from build123d import *

# Parameters (mm, degrees)
SKETCH1_R           = 5.08
BOSS_EXTRUDE1_DEPTH = 20.8
SKETCH2_R           = 10.16
BOSS_EXTRUDE2_DEPTH = 13.97
SKETCH4_R           = 6.052157879
SKETCH3_R           = 6.450000054
CHAMFER1_SIZE       = 5.08


with BuildPart() as part:
    # Sketch1 → Boss-Extrude1 (new body)
    with BuildSketch(Plane(origin=(0, 0, 0), x_dir=(1, 0, 0), z_dir=(0, 1, 0))):
        with Locations(Location((0, 0, 0), (0, 0, 270))):
            Circle(SKETCH1_R)
    extrude(amount=BOSS_EXTRUDE1_DEPTH)

    # Sketch2 → Boss-Extrude2 (add)
    with BuildSketch(Plane(origin=(0, 20.8, 0), x_dir=(1, 0, 0), z_dir=(0, 1, 0))):
        with Locations(Location((0, 0, 0), (0, 0, 270))):
            Circle(SKETCH2_R)
    extrude(amount=BOSS_EXTRUDE2_DEPTH)

    # Sketch4 → Cut-Loft1 section 0
    with BuildSketch(Plane(origin=(0, 23.34, 0), x_dir=(-1, 0, 0), z_dir=(0, -1, 0))):
        Circle(SKETCH4_R)
    # Sketch3 → Cut-Loft1 section 1
    with BuildSketch(Plane(origin=(0, 34.77, 0), x_dir=(1, 0, 0), z_dir=(0, 1, 0))):
        Circle(SKETCH3_R)
    loft(mode=Mode.SUBTRACT)

    # Chamfer1
    chamfer1_edges = [part.edges().sort_by_distance(p)[0] for p in [
        (0, 20.8, -5.08),
    ]]
    chamfer(chamfer1_edges, length=CHAMFER1_SIZE - 0.0001)  # a hair under: the kernel refuses the full size

    # Cut-Loft2: read off the stored shape, not the designer's step
    # Cut-Loft2: loft between two sections, ruled curve by curve
    cut_loft2_from = [
        Edge.make_bspline([(-1.686897944, 18.26, -1.600000102), (-1.546323115, 18.26, -1.600000102), (-1.405748287, 18.26, -1.600000102), (-1.124598629, 18.26, -1.600000102), (-0.984023801, 18.26, -1.600000102), (-0.702874143, 18.26, -1.600000102), (-0.562299315, 18.26, -1.600000102), (-0.281149657, 18.26, -1.600000102), (-0.140574829, 18.26, -1.600000102), (0.140574829, 18.26, -1.600000102), (0.281149657, 18.26, -1.600000102), (0.562299315, 18.26, -1.600000102), (0.702874143, 18.26, -1.600000102), (0.984023801, 18.26, -1.600000102), (1.124598629, 18.26, -1.600000102), (1.405748287, 18.26, -1.600000102), (1.546323115, 18.26, -1.600000102), (1.686897944, 18.26, -1.600000102)], [0, 0, 0, 0, 0.125, 0.125, 0.25, 0.25, 0.375, 0.375, 0.5, 0.5, 0.625, 0.625, 0.75, 0.75, 0.875, 0.875, 1, 1, 1, 1], 3),
        Edge.make_bspline([(1.686897944, 18.26, -1.600000102), (3.329599086, 18.26, 0.131918024), (2.387049944, 18.26, 2.325), (-2.387049944, 18.26, 2.325), (-3.329599086, 18.26, 0.131918024), (-1.686897944, 18.26, -1.600000102)], [0, 0, 0, 0, 0.5, 0.5, 1, 1, 1, 1], 3, [1, 0.355899276, 0.212319878, 0.212319878, 0.355899276, 1]),
    ]
    cut_loft2_to = [
        Edge.make_bspline([(-2.182602074, 0, -1.269595679), (-2.091149197, 0, -1.426815211), (-1.976752522, 0, -1.584210464), (-1.696673404, 0, -1.88110943), (-1.530809339, 0, -2.020452874), (-1.151990541, 0, -2.25799133), (-0.939007592, 0, -2.355871773), (-0.483917032, 0, -2.489516293), (-0.242057859, 0, -2.525), (0.242057859, 0, -2.525), (0.483917032, 0, -2.489516293), (0.939007592, 0, -2.355871773), (1.151990541, 0, -2.25799133), (1.530809339, 0, -2.020452874), (1.696673404, 0, -1.88110943), (1.976752522, 0, -1.584210464), (2.091149197, 0, -1.426815211), (2.182602074, 0, -1.269595679)], [0, 0, 0, 0, 0.125, 0.125, 0.25, 0.25, 0.375, 0.375, 0.5, 0.5, 0.625, 0.625, 0.75, 0.75, 0.875, 0.875, 1, 1, 1, 1], 3),
        Edge.make_bspline([(2.182602074, 0, -1.269595679), (3.284684333, 0, 0.625028778), (2.191845601, 0, 2.525), (-2.191845601, 0, 2.525), (-3.284684333, 0, 0.625028778), (-2.182602074, 0, -1.269595679)], [0, 0, 0, 0, 0.5, 0.5, 1, 1, 1, 1], 3, [1, 0.4431946, 0.295047331, 0.295047331, 0.4431946, 1]),
    ]
    cut_loft2 = Solid(Shell([*[Face.make_surface_from_curves(cut_loft2_from[k], cut_loft2_to[k]) for k in range(2)], Face(Wire(cut_loft2_from)), Face(Wire(cut_loft2_to))]))
    add(cut_loft2, mode=Mode.SUBTRACT)


solid = part.part
Geometry check sheet. Reference: the model listing, model coordinates, mm. A direction names the side the tool comes from. Give positions to 0.01 mm unless a question says otherwise; leave off trailing zeros. Loops run counter-clockwise (first coordinate to the right, second up) from the corner with the lowest first, then second, coordinate; pieces in that order, holes last. Notation, with made-up numbers: M 10.5,61.5 L 17.5,61.5 A30 cw 17.5,84.5 Z; hole C 81.5,-5 d9. An arc over 180 degrees is marked long. Write each question's results on one line, items separated by ' | '.
1) Tool access check on faces 4 (the face through (-7, 34.77, 0)), 5 (the face through (0, 23.34, 0)), 6 (the face through (5.037, 7.75, -0.661)). Record the directions out of +Z, -Z, +X, -X, +Y, -Y that give a thin tool (end or side, any length) a straight path to the whole face; none if there is none.
Answers follow:
face 4: +Z, -Z, +X, -X, +Y | face 5: +Y | face 6: -Y
2) Thickness scan on line 1 (Y direction, x = 1.75, z = 0.5); line 2 (Y direction, x = -3, z = 1.75); line 3 (X direction, y = 26, z = -2.75). Record the ranges inside material, lowest first.
Answers follow:
line 1: 18.26 to 23.34 | line 2: 0 to 23.34 | line 3: -9.78 to -5.5, 5.5 to 9.78
3) Gauge pin test, flat ends, axial feed: pin 1 (1 mm diameter, centred on x = -1.5, z = 0, fed in from -Y); pin 2 (1 mm diameter, centred on x = -7.5, z = -4.5, fed in from -Y); pin 3 (1 mm diameter, centred on x = 0.5, y = 10.5, fed in from -Z). Record the tip position at first contact, or that the pin passes through.
Answers follow:
pin 1: y = 18.26 | pin 2: y = 18.89 | pin 3: z = -5.08
4) Section check A-A, the plane y = 30. Record the boundary of the cut face in (x, z), plus the area to 3 significant figures.
Answers follow:
outline: C 0,0 d20.32; hole C 0,0 d12.57 | area: 200 mm2
5) Release check for a two-part mould opening along X. For faces 1 (the face through (0, 18.26, 0)), 2 (the face through (-2, 0, 2)), 3 (the face through (10.074, 27.687, -1.323)) record: +X half, -X half, draft (parallel to the pull), parting line (faces both ways), or undercut.
Answers follow:
face 1: undercut | face 2: draft | face 3: parting line
